Verification items for the finished model (mm, model axes). Face numbers are marked on the shaded views. Coordinates: 2 decimals unless noted, no trailing zeros. Write each loop counter-clockwise with the first axis right and the second up, starting at its lowest first coordinate (ties: lowest second). Pieces come first, ordered by that corner, then holes. Notation, with made-up numbers: M 41.25,-24.75 L 60.25,-24.75 A13 ccw 60.25,-8.75 Z; hole C 20,69 d3. An arc over 180 degrees is marked long. One line per item, written item: value.
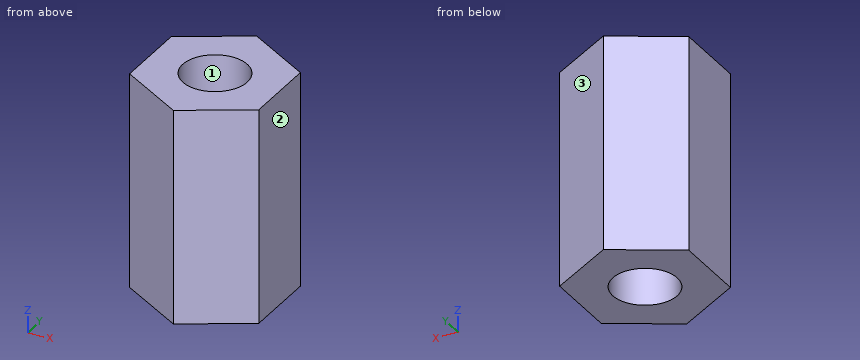
Autodesk Inventor part; units mm, degrees
ref_plane "YZ Plane" through (0, 0, 0) normal (1, 0, 0) x (0, 1, 0)
ref_plane "XZ Plane" through (0, 0, 0) normal (0, 1, 0) x (-1, 0, 0)
ref_plane "XY Plane" through (0, 0, 0) normal (0, 0, 1) x (1, 0, 0)
sketch "Эскиз1" plane through (0, 0, 0) normal (0, 0, 1) x (1, 0, 0)
  line L0 (0, 3.4641) -> (3, 1.7321)
  line L1 (3, 1.7321) -> (3, -1.7321)
  line L2 (3, -1.7321) -> (0, -3.4641)
  line L3 (0, -3.4641) -> (-3, -1.7321)
  line L4 (-3, -1.7321) -> (-3, 1.7321)
  line L5 (-3, 1.7321) -> (0, 3.4641)
  circle A0 centre (0, 0) radius 1.5
  dimension "d0" = 3
  dimension "d1" = 6
extrude "Выдавливание1" add sketch "Эскиз1" along normal mid plane 10
properties part number "Стойка м3х10"
Item 1: Cross-section at C-C, the plane x = -0.5. Enter the section's corners in (y, z), and give its area (3 significant figures).
The answers:
outline: M -3.18,-5 L -1.41,-5 L -1.41,5 L -3.18,5 Z; M 1.41,-5 L 3.18,-5 L 3.18,5 L 1.41,5 Z
area: 35.2 mm²
Item 2: Cross-section at A-A, the plane y = 0. Enter the section's corners in (x, z), and give its area (3 significant figures).
The answers:
outline: M -3,-5 L -1.5,-5 L -1.5,5 L -3,5 Z; M 1.5,-5 L 3,-5 L 3,5 L 1.5,5 Z
area: 30.0 mm²
Item 3: Cross-section at B-B, the plane z = -3.5. Enter the section's corners in (x, y).
The answers:
outline: M -3,-1.73 L 0,-3.46 L 3,-1.73 L 3,1.73 L 0,3.46 L -3,1.73 Z; hole C 0,0 d3
Item 4: Scan lines: line 1 (Y direction, x = 0.6, z = 2.75); line 2 (X direction, y = 1.25, z = 0); line 3 (Y direction, x = -0.3, z = -4). Record each from-to range of solid material in increasing order.
The answers:
line 1: y = -3.12 to -1.37, 1.37 to 3.12
line 2: x = -3 to -0.83, 0.83 to 3
line 3: y = -3.29 to -1.47, 1.47 to 3.29
Item 5: Cross-section at D-D, the plane y = 2.75. Enter the section's corners in (x, z).
The answers:
outline: M -1.24,-5 L 1.24,-5 L 1.24,5 L -1.24,5 Z
Item 6: Draft check along Y on the marked faces 1, 2 and 3. Enter one of: released by +Y, released by -Y, zero draft, split by the parting line, or undercut.
The answers:
face 1: undercut
face 2: zero draft
face 3: released by +Y
